Build history of the part. All positions in model axes, mm. Face numbers are marked on the shaded views. Give positions to 0.01 mm unless a question says otherwise; leave off trailing zeros. Order: outer loops, then holes, each group sorted by start corner. A loop starts at its lowest first (then second) coordinate and runs counter-clockwise, first axis right, second up. Notation, with made-up numbers: (51.5, -12.5) - (92.5, -12.5) arc R26 cw to (92.5, 6.5) - close; hole circle Ø7 at (66, 7). An arc over 180 degrees is marked (long way). One line per item, written item: value.
```python
from build123d import *

# Parameters (mm, degrees)
SZKIC1_R                        = 30
DODANIE_WYCI_GNI_CIE1_DEPTH     = 40
WYTNIJ_WYCI_GNI_CIE1_DEPTH      = 59.309518948
WYTNIJ_WYCI_GNI_CIE1_DEPTH_BACK = 59.309518948
SZKIC4_R                        = 10
WYTNIJ_WYCI_GNI_CIE2_DEPTH      = 2


with BuildPart() as part:
    # Szkic1 → Dodanie-wyciągnięcie1 (new body)
    with BuildSketch(Plane.XY):
        Circle(SZKIC1_R)
    extrude(amount=DODANIE_WYCI_GNI_CIE1_DEPTH)

    # Szkic2 → Wytnij-wyciągnięcie1 (cut, two sides: drawn at the far end of the back side and taken through both)
    with BuildSketch(Plane(origin=(0, 0, 0), x_dir=(0, 0, -1), z_dir=(1, 0, 0)).offset(-WYTNIJ_WYCI_GNI_CIE1_DEPTH_BACK)):
        with BuildLine():
            ThreePointArc((-19.746856725, 0), (-25.463814718, 15.911137324), (-40, 24.545210352))
            Line((-40, 24.545210352), (-40, -24.545210352))
            ThreePointArc((-40, -24.545210352), (-25.463814718, -15.911137324), (-19.746856725, 0))
        make_face()
        with BuildLine():
            Line((-40, -24.545210352), (-40, 24.545210352))
            ThreePointArc((-40, 24.545210352), (-69.746856725, 0), (-40, -24.545210352))
        make_face()
    extrude(amount=WYTNIJ_WYCI_GNI_CIE1_DEPTH + WYTNIJ_WYCI_GNI_CIE1_DEPTH_BACK, mode=Mode.SUBTRACT)

    # Szkic4 → Wytnij-wyciągnięcie2 (cut)
    with BuildSketch(Plane(origin=(0, 0, 0), x_dir=(-1, 0, 0), z_dir=(0, 0, -1))):
        Circle(SZKIC4_R)
    extrude(amount=-WYTNIJ_WYCI_GNI_CIE2_DEPTH, mode=Mode.SUBTRACT)


solid = part.part
```
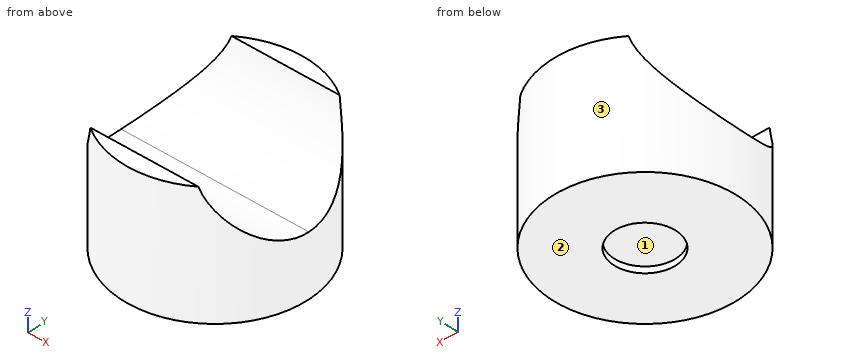
(1) Slice it at A-A, the plane x = 0. Give the cut face in (y, z), and give its area (3 significant figures).
Completed:
outline: (-30, 0) - (-10, 0) - (-10, 2) - (10, 2) - (10, 0) - (30, 0) - (30, 40) - (24.55, 40) arc R25 cw to (-24.55, 40) - (-30, 40) - close
area: 1,610 mm²
(2) Drill centre lines: line 1 (Y direction, x = 0, z = 0.9); line 2 (Y direction, x = -3, z = 22); line 3 (Z direction, x = 19, y = -0.5). Where is each one in solid material? Low to high.
Completed:
line 1: -30 to -10, 10 to 30
line 2: -29.85 to -10.37, 10.37 to 29.85
line 3: 0 to 19.75
(3) Slice it at C-C, the plane x = 12.5. Give the cut face in (y, z), and give its area (3 significant figures).
Completed:
outline: (-27.27, 0) - (27.27, 0) - (27.27, 40) - (24.55, 40) arc R25 cw to (-24.55, 40) - (-27.27, 40) - close
area: 1,440 mm²
(4) Slice it at D-D, the plane z = 6.5. Give the cut face in (x, y), and give its area (3 significant figures).
Completed:
outline: circle Ø60 at (0, 0)
area: 2,830 mm²
(5) Pin check, flat tips, straight feed: P1, Ø6, axis at x = 8.5, z = 18, coming from the +Y side; P2, Ø23, axis at x = 0, y = 0, coming from the +Z side; P3, Ø3, axis at x = -9, z = 12.5, coming from the +Y side. Stop position of each tip, or through.
Completed:
P1: y = 29.49
P2: z = 22.55
P3: y = 29.05
(6) Slice it at B-B, the plane z = 36.5. Give the cut face in (x, y).
Completed:
outline: (-18.52, -23.6) arc R30 ccw to (18.52, -23.6) - close; (-18.52, 23.6) - (18.52, 23.6) arc R30 ccw to start
(7) Pull direction Y, two halves, no side cores. Call the marked faces 1, 2 and 3: +Y half, -Y half, draft (parallel to the pull), parting line (faces both ways), or undercut.
Completed:
face 1: undercut
face 2: draft
face 3: parting line
